Design review of the part built by this model. Coordinates are the model's own, in mm. Face numbers are marked on the shaded views. A direction names the side the tool comes from. Coordinates: 2 decimals unless noted, no trailing zeros. Write each loop counter-clockwise with the first axis right and the second up, starting at its lowest first coordinate (ties: lowest second). Pieces come first, ordered by that corner, then holes.
Q1. Insertion check: pin 1 (12 mm diameter, centred on x = 0, z = 2.5, fed in from -Y). The pin has a flat end and moves straight along its axis. Give the tip position at first contact, or say it passes through.
Q2. Machinability: for the marked faces 1 and 2, which of the approach directions +Z, -Z, +X, -X, +Y, -Y give a long, thin tool a straight path to every point of the face, cutting with its end or side? Answer none if there is none.
Q3. For probe 1 along Z at (x, y) = (-15, 0.9) (3 decimals); probe 2 along X at (y, z) = (2.2, 3.5); probe 3 along Z at (x, y) = (-24, 1.7), list the stretches that pass through material, from the lowest coordinate up.
Q4. Take a section at A-A (y = 3.65). Give the boundary of the cut face in (x, z) (3 decimals).
Q5. Take a section at B-B (z = 5). Give the boundary of the cut face in (x, y), and give its area (3 significant figures).
Q6. Take a section at D-D (z = -8.5). Give the boundary of the cut face in (x, y).
Q7. Mouldability with a two-part tool opening along X and no side actions: class the marked faces 3, 4, 5 and 6 as pulls with the +X half, pulls with the -X half, needs draft (parallel to the pull), parting line crosses it, or undercut.
Q8. Take a section at C-C (x = 17). Give the boundary of the cut face in (y, z) (3 decimals).
```python
from build123d import *

# Parameters (mm, degrees)
SKETCH1_W                  = 55.620000012
SKETCH1_H                  = 27.550000018
SKETCH1_W_2                = 41.29999995
SKETCH1_H_2                = 21.200000018
BOSS_EXTRUDE1_DEPTH        = 5.1308
F_4_9_4_9_DIAMETER_HOLE1_D = 4.9
FILLET1_R                  = 6.35
FILLET2_R                  = 1.27


with BuildPart() as part:
    # Sketch1 → Boss-Extrude1 (new body)
    with BuildSketch(Plane(origin=(0, 0, 0), x_dir=(1, 0, 0), z_dir=(0, 1, 0))):
        Rectangle(SKETCH1_W, SKETCH1_H)
        Rectangle(SKETCH1_W_2, SKETCH1_H_2, mode=Mode.SUBTRACT)
    extrude(amount=BOSS_EXTRUDE1_DEPTH)

    # Ø4.9 (4.9) Diameter Hole1 (through all)
    with Locations(Plane(origin=(0, 5.1308, 0), x_dir=(1, 0, 0), z_dir=(0, 1, 0))):
        with Locations((24, -5), (-24, 5), (-24, -5), (24, 5)):
            Hole(F_4_9_4_9_DIAMETER_HOLE1_D / 2)

    # Fillet1
    fillet1_edges = [part.edges().sort_by_distance(p)[0] for p in [
        (27.810000006, 2.5654, 13.775000009),
        (-27.810000006, 2.5654, 13.775000009),
        (-27.810000006, 2.5654, -13.775000009),
        (27.810000006, 2.5654, -13.775000009),
    ]]
    fillet(fillet1_edges, radius=FILLET1_R)

    # Fillet2
    fillet2_edges = [part.edges().sort_by_distance(p)[0] for p in [
        (20.649999975, 2.5654, 10.600000009),
        (20.649999975, 2.5654, -10.600000009),
        (-20.649999975, 2.5654, -10.600000009),
        (-20.649999975, 2.5654, 10.600000009),
    ]]
    fillet(fillet2_edges, radius=FILLET2_R)


solid = part.part
```
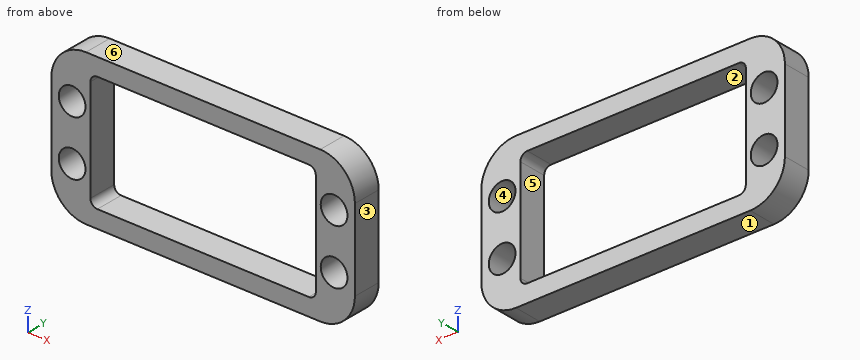
Response:
1. pin 1: passes through
2. face 1: -Z, +X, -X, +Y, -Y
2. face 2: +Y, -Y
3. probe 1: z = -13.775 to -10.6, 10.6 to 13.775
3. probe 2: x = -27.81 to -25.94, -22.06 to -20.65, 20.65 to 22.06, 25.94 to 27.81
3. probe 3: z = -13.24 to -7.45, -2.55 to 2.55, 7.45 to 13.24
4. outline: (-27.81, -7.425) arc R6.35 ccw to (-21.46, -13.775) - (21.46, -13.775) arc R6.35 ccw to (27.81, -7.425) - (27.81, 7.425) arc R6.35 ccw to (21.46, 13.775) - (-21.46, 13.775) arc R6.35 ccw to (-27.81, 7.425) - close; hole circle Ø4.9 at (-24, -5); hole circle Ø4.9 at (-24, 5); hole (-20.65, -9.33) arc R1.27 ccw to (-19.38, -10.6) - (19.38, -10.6) arc R1.27 ccw to (20.65, -9.33) - (20.65, 9.33) arc R1.27 ccw to (19.38, 10.6) - (-19.38, 10.6) arc R1.27 ccw to (-20.65, 9.33) - close; hole circle Ø4.9 at (24, -5); hole circle Ø4.9 at (24, 5)
5. outline: (-27.81, 0) - (-26.45, 0) - (-26.45, 5.13) - (-27.81, 5.13) - close; (-21.55, 0) - (-20.65, 0) - (-20.65, 5.13) - (-21.55, 5.13) - close; (20.65, 0) - (21.55, 0) - (21.55, 5.13) - (20.65, 5.13) - close; (26.45, 0) - (27.81, 0) - (27.81, 5.13) - (26.45, 5.13) - close
5. area: 23.2 mm2
6. outline: (-27.72, 0) - (-20.65, 0) - (-20.65, 5.13) - (-27.72, 5.13) - close; (20.65, 0) - (27.72, 0) - (27.72, 5.13) - (20.65, 5.13) - close
7. face 3: pulls with the +X half
7. face 4: undercut
7. face 5: undercut
7. face 6: needs draft
8. outline: (0, -13.775) - (5.131, -13.775) - (5.131, -10.6) - (0, -10.6) - close; (0, 10.6) - (5.131, 10.6) - (5.131, 13.775) - (0, 13.775) - close
